Verification items for the finished model (mm, model axes). A direction names the side the tool comes from. Coordinates: 2 decimals unless noted, no trailing zeros. Order: outer loops, then holes, each group sorted by start corner. A loop starts at its lowest first (then second) coordinate and runs counter-clockwise, first axis right, second up. Notation, with made-up numbers: M -16,-24 L -5,-24 A30 cw -5,9 Z; hole C 88.5,53 d4. An arc over 180 degrees is marked long. Write item = value, one per line.
```python
from build123d import *

# Parameters (mm, degrees)
SKETCH1_W           = 39
SKETCH1_H           = 13
SKETCH1_R           = 1.4
BOSS_EXTRUDE2_DEPTH = 7.5
SKETCH2_R           = 1.75
CUT_EXTRUDE1_DEPTH  = 26.615367173
CUT_EXTRUDE2_DEPTH  = 0.5


with BuildPart() as part:
    # Sketch1 → Boss-Extrude2 (new body)
    with BuildSketch(Plane.XY):
        with Locations((1.258059529, -6.888438134)):
            Rectangle(SKETCH1_W, SKETCH1_H)
        with Locations((-15.091940471, -10.238438134)):
            Circle(SKETCH1_R, mode=Mode.SUBTRACT)
        with Locations((17.608059529, -10.238438134)):
            Circle(SKETCH1_R, mode=Mode.SUBTRACT)
    extrude(amount=-BOSS_EXTRUDE2_DEPTH)

    # Sketch2 → Cut-Extrude1 (cut, through all)
    with BuildSketch(Plane(origin=(0, -0.388438134, 0), x_dir=(1, 0, 0), z_dir=(0, 1, 0))):
        with Locations(Location((-11.241940471, 3.75, 0), (0, 0, 180))):
            Circle(SKETCH2_R)
        with Locations(Location((13.758059529, 3.75, 0), (0, 0, 180))):
            Circle(SKETCH2_R)
    extrude(amount=-CUT_EXTRUDE1_DEPTH, mode=Mode.SUBTRACT)

    # Sketch3 → Cut-Extrude2 (cut)
    with BuildSketch(Plane.XY):
        with BuildLine():
            Line((-1.789484561, -4.361984997), (0.528429434, -4.361984997))
            ThreePointArc((0.528429434, -4.361984997), (2.118216576, -5.694764696), (0.528429434, -7.027544395))
            Line((0.528429434, -7.027544395), (-0.758815547, -7.027544395))
            ThreePointArc((-0.758815547, -7.027544395), (-0.847047418, -7.240554977), (-0.758815547, -7.453565558))
            Line((-0.758815547, -7.453565558), (1.285636155, -7.453565558))
            ThreePointArc((1.285636155, -7.453565558), (2.238737943, -8.66797631), (1.168769854, -9.780794705))
            Line((1.168769854, -9.780794705), (-1.789484561, -9.780794705))
            Line((-1.789484561, -9.780794705), (-1.789484561, -4.361984997))
        make_face()
        with BuildLine():
            Line((-1.006496381, -4.819305585), (-1.006496381, -6.678234448))
            Line((-1.006496381, -6.678234448), (0.528429434, -6.678234448))
            ThreePointArc((0.528429434, -6.678234448), (1.377263921, -5.748770016), (0.528429434, -4.819305585))
            Line((0.528429434, -4.819305585), (-1.006496381, -4.819305585))
        make_face(mode=Mode.SUBTRACT)
        with BuildLine():
            Line((-1.006496381, -7.858595879), (-1.006496381, -9.373009321))
            Line((-1.006496381, -9.373009321), (0.528429434, -9.373009321))
            ThreePointArc((0.528429434, -9.373009321), (1.285636155, -8.6158026), (0.528429434, -7.858595879))
            Line((0.528429434, -7.858595879), (-1.006496381, -7.858595879))
        make_face(mode=Mode.SUBTRACT)
    extrude(amount=-CUT_EXTRUDE2_DEPTH, mode=Mode.SUBTRACT)


solid = part.part
```
Item 1: Tool access check on faces 1 (the flat face through (-18.242, -7, -4)), 2 (the cylindrical face through (2.118, -5.662, -0.246)). Record the directions out of +Z, -Z, +X, -X, +Y, -Y that give a thin tool (end or side, any length) a straight path to the whole face; none if there is none.
Report:
face_1 = +Z, -Z, -X, +Y, -Y
face_2 = +Z
Item 2: Sectioned sample at C-C, the plane y = -2. Enter the section's corners in (x, z), then the cut area to 3 significant figures.
Report:
outline = M -18.24,-7.5 L 20.76,-7.5 L 20.76,0 L -18.24,0 Z; hole C -11.24,-3.75 d3.5; hole C 13.76,-3.75 d3.5
area = 273 mm^2
Item 3: Sectioned sample at D-D, the plane x = 15. Enter the section's corners in (y, z), then the cut area to 3 significant figures.
Report:
outline = M -13.39,-7.5 L -0.39,-7.5 L -0.39,-4.98 L -13.39,-4.98 Z; M -13.39,-2.52 L -0.39,-2.52 L -0.39,0 L -13.39,0 Z
area = 65.4 mm^2
Item 4: Sectioned sample at B-B, the plane y = -11. Enter the section's corners in (x, z), then the cut area to 3 significant figures.
Report:
outline = M -18.24,-7.5 L -16.27,-7.5 L -16.27,0 L -18.24,0 Z; M -13.92,-7.5 L 16.43,-7.5 L 16.43,0 L -13.92,0 Z; M 18.78,-7.5 L 20.76,-7.5 L 20.76,0 L 18.78,0 Z; hole C -11.24,-3.75 d3.5; hole C 13.76,-3.75 d3.5
area = 238 mm^2
Item 5: Sectioned sample at A-A, the plane z = -3.75. Enter the section's corners in (x, y).
Report:
outline = M -18.24,-13.39 L -12.99,-13.39 L -12.99,-0.39 L -18.24,-0.39 Z; M -9.49,-13.39 L 12.01,-13.39 L 12.01,-0.39 L -9.49,-0.39 Z; M 15.51,-13.39 L 20.76,-13.39 L 20.76,-0.39 L 15.51,-0.39 Z; hole C -15.09,-10.24 d2.8; hole C 17.61,-10.24 d2.8
Item 6: Scan lines: L1, parallel to X at y = -10.25, z = -7; L2, parallel to X at y = -2.75, z = -2.75; L3, parallel to Y at x = -14.5, z = -5.5. Record each from-to range of solid material in increasing order. Write a range as from..to.
Report:
L1 = -18.24..-16.49, -13.69..16.21, 19.01..20.76
L2 = -18.24..-12.68, -9.81..12.32, 15.19..20.76
L3 = -13.39..-11.51, -8.97..-0.39
Item 7: Release check for a two-part mould opening along X. For faces 3 (the cylindrical face through (-16.12, -9.29, -3.7)), 4 (the flat face through (1, -13.388, -4)), 5 (the flat face through (20.758, -7, -4)) record: pulls with the +X half, pulls with the -X half, needs draft (parallel to the pull), parting line crosses it, or undercut.
Report:
face_3 = undercut
face_4 = needs draft
face_5 = pulls with the +X half
